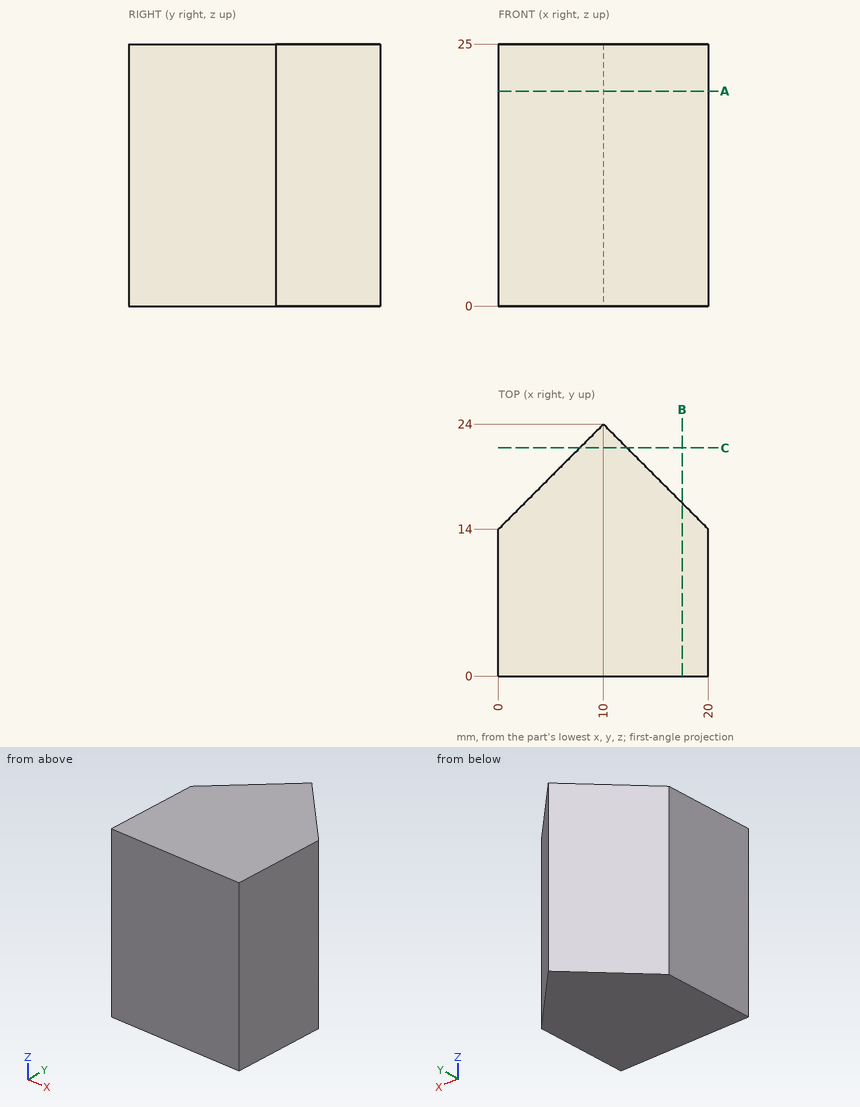
Part print with two shaded views. Sizes in mm from the minimum x, y, z corner. Round coordinates to 2 decimals unless told otherwise and drop trailing zeros. Order: outer loops, then holes, each group sorted by start corner. A loop starts at its lowest first (then second) coordinate and runs counter-clockwise, first axis right, second up. Notation, with made-up numbers: (84, -28.5) - (140, -28.5) arc R16 ccw to (140, -22.5) - close; hole circle Ø3 at (-30, 13). An arc over 180 degrees is marked (long way). Answer in a Markdown table with one row per item. Add a question column.
(1) Band-saw the part on B-B on x = 17.5. List the corners of the cut face in (y, z).
(2) Band-saw the part on A-A on z = 20.5. List the corners of the cut face in (x, y), and give its area (3 significant figures).
(3) Band-saw the part on C-C on y = 21.75. List the corners of the cut face in (x, z).
(4) Probe L1, parallel to Y at x = 18.25, z = 7; L2, parallel to X at y = 20.25, z = 21.75; L3, parallel to Y at x = 8.5, z = 22. List the from-to ranges inside material, lowest first. Write a range as [from, to].
(5) Drop a flat-ended pin along its axis: pin 1 Ø1.5 at (x, z) = (16.5, 19.5) entering from +Y. Give the stop position or say it passes through.
Data:
| question | item | result |
|---|---|---|
| 1 | outline | (0, 0) - (16.5, 0) - (16.5, 25) - (0, 25) - close |
| 2 | outline | (0, 0) - (20, 0) - (20, 14) - (10, 24) - (0, 14) - close |
| 2 | area | 380 mm^2 |
| 3 | outline | (7.75, 0) - (12.25, 0) - (12.25, 25) - (7.75, 25) - close |
| 4 | L1 | y = [0, 15.75] |
| 4 | L2 | x = [6.25, 13.75] |
| 4 | L3 | y = [0, 22.5] |
| 5 | pin 1 | stops at y = 18.25 |
